Could you check a few things on this model? Use its own coordinates, in mm. A direction names the side the tool comes from. Give positions to 0.01 mm unless a question says otherwise; leave off trailing zeros. Write each loop counter-clockwise with the first axis right and the second up, starting at its lowest first coordinate (ties: lowest second). Pieces come first, ordered by that corner, then holes. Notation, with made-up numbers: (57.5, -14.75) - (90.5, -14.75) arc R13 ccw to (90.5, -4.75) - close; hole circle Ø10 at (20.5, 32). An arc over 180 degrees is marked (long way). Write item = value, one per line.
from build123d import *

# Parameters (mm, degrees)
BOSS_EXTRUDE1_DEPTH = 60
CUT_EXTRUDE3_REACH  = 29
SKETCH8_R           = 3.999999996
CUT_EXTRUDE4_REACH  = 52
SKETCH9_R           = 4.000000003
FILLET2_R           = 2


with BuildPart() as part:
    # Sketch1 → Boss-Extrude1 (new body)
    with BuildSketch(Plane(origin=(0, 0, 0), x_dir=(0, 0, -1), z_dir=(1, 0, 0))):
        Polygon((0, 0), (0, 50), (4, 50), (4, 4), (27, 4), (27, 0), align=None)
    extrude(amount=BOSS_EXTRUDE1_DEPTH)

    # Sketch8 → Cut-Extrude3 (cut, up to next)
    with BuildSketch(Plane.XY, mode=Mode.PRIVATE) as cut_extrude3_sk1:
        with Locations((10, 22)):
            Circle(SKETCH8_R)
    cut_extrude3_tool1 = extrude(cut_extrude3_sk1.sketch, amount=-CUT_EXTRUDE3_REACH, mode=Mode.PRIVATE) & part.part
    add(cut_extrude3_tool1.solids().sort_by_distance((10, 22, 0))[0], mode=Mode.SUBTRACT)
    # Sketch8 → Cut-Extrude3 (cut, up to next)
    with BuildSketch(Plane.XY, mode=Mode.PRIVATE) as cut_extrude3_sk2:
        with Locations((50, 22)):
            Circle(SKETCH8_R)
    cut_extrude3_tool2 = extrude(cut_extrude3_sk2.sketch, amount=-CUT_EXTRUDE3_REACH, mode=Mode.PRIVATE) & part.part
    add(cut_extrude3_tool2.solids().sort_by_distance((50, 22, 0))[0], mode=Mode.SUBTRACT)
    # Sketch8 → Cut-Extrude3 (cut, up to next)
    with BuildSketch(Plane.XY, mode=Mode.PRIVATE) as cut_extrude3_sk3:
        with Locations((50, 42)):
            Circle(SKETCH8_R)
    cut_extrude3_tool3 = extrude(cut_extrude3_sk3.sketch, amount=-CUT_EXTRUDE3_REACH, mode=Mode.PRIVATE) & part.part
    add(cut_extrude3_tool3.solids().sort_by_distance((50, 42, 0))[0], mode=Mode.SUBTRACT)
    # Sketch8 → Cut-Extrude3 (cut, up to next)
    with BuildSketch(Plane.XY, mode=Mode.PRIVATE) as cut_extrude3_sk4:
        with Locations((10, 42)):
            Circle(SKETCH8_R)
    cut_extrude3_tool4 = extrude(cut_extrude3_sk4.sketch, amount=-CUT_EXTRUDE3_REACH, mode=Mode.PRIVATE) & part.part
    add(cut_extrude3_tool4.solids().sort_by_distance((10, 42, 0))[0], mode=Mode.SUBTRACT)

    # Sketch9 → Cut-Extrude4 (cut, up to next)
    with BuildSketch(Plane.XZ, mode=Mode.PRIVATE) as cut_extrude4_sk1:
        with Locations((50, -19)):
            Circle(SKETCH9_R)
    cut_extrude4_tool1 = extrude(cut_extrude4_sk1.sketch, amount=-CUT_EXTRUDE4_REACH, mode=Mode.PRIVATE) & part.part
    add(cut_extrude4_tool1.solids().sort_by_distance((50, 0, -19))[0], mode=Mode.SUBTRACT)
    # Sketch9 → Cut-Extrude4 (cut, up to next)
    with BuildSketch(Plane.XZ, mode=Mode.PRIVATE) as cut_extrude4_sk2:
        with Locations((10, -19)):
            Circle(SKETCH9_R)
    cut_extrude4_tool2 = extrude(cut_extrude4_sk2.sketch, amount=-CUT_EXTRUDE4_REACH, mode=Mode.PRIVATE) & part.part
    add(cut_extrude4_tool2.solids().sort_by_distance((10, 0, -19))[0], mode=Mode.SUBTRACT)

    # Fillet2
    fillet2_edges = [part.edges().sort_by_distance(p)[0] for p in [
        (60, 50, -2),
        (0, 50, -2),
        (60, 2, -27),
        (0, 2, -27),
    ]]
    fillet(fillet2_edges, radius=FILLET2_R)


solid = part.part
1. I need wall thicknesses on line 1 (Z direction, x = 10, y = 2.4); line 2 (X direction, y = 39, z = -2.25); line 3 (Z direction, x = 37, y = 19). Which ranges of each line are inside material? Lowest first, please.
Filled sheet:
line_1 = -27 to -23, -15 to 0
line_2 = 0 to 7.35, 12.65 to 47.35, 52.65 to 60
line_3 = -4 to 0
2. For pin 1 (6.5 mm diameter, centred on x = 50, y = 22, fed in from +Z); pin 2 (11.5 mm diameter, centred on x = 35, z = -18, fed in from +Y); pin 3 (4 mm diameter, centred on x = 10.5, y = 37.5, fed in from -Z), each with a flat end and sliding along its axis, tell me the tip position at first contact or that it passes through.
Filled sheet:
pin_1 = through
pin_2 = 4
pin_3 = -4
3. Thinking about a two-plate mould opening in Z: for faces 3 (the face through (13.815, 1.972, -17.799)), 4 (the face through (60, 17, -3)), 5 (the face through (30, 25, 0)), which applies, pulls with the +Z half, pulls with the -Z half, needs draft (parallel to the pull), parting line crosses it, or undercut?
Filled sheet:
face_3 = undercut
face_4 = needs draft
face_5 = pulls with the +Z half
4. If we section it at D-D, the plane x = 33: Please give me the cut outline in (y, z).
Filled sheet:
outline = (0, -27) - (4, -27) - (4, -4) - (50, -4) - (50, 0) - (0, 0) - close
5. Which directions (+Z, -Z, +X, -X, +Y, -Y) give clear straight access to the entire face, cutting with the end or side of a thin tool? Please do faces 1 (the face through (30, 27, -4)), 2 (the face through (30, 0, -14)).
Filled sheet:
face_1 = -Z, +X, -X, +Y
face_2 = +Z, -Z, +X, -X, -Y
6. If we section it at A-A, the plane z = -19: Please give me the cut outline in (x, y), and give its area (3 significant figures).
Filled sheet:
outline = (0, 0) - (6, 0) - (6, 4) - (0, 4) - close; (14, 0) - (46, 0) - (46, 4) - (14, 4) - close; (54, 0) - (60, 0) - (60, 4) - (54, 4) - close
area = 176 mm2
7. If we section it at C-C, the plane y = 22: Please give me the cut outline in (x, z), and give its area (3 significant figures).
Filled sheet:
outline = (0, -4) - (6, -4) - (6, 0) - (0, 0) - close; (14, -4) - (46, -4) - (46, 0) - (14, 0) - close; (54, -4) - (60, -4) - (60, 0) - (54, 0) - close
area = 176 mm2
8. If we section it at B-B, the plane x = 10: Please give me the cut outline in (y, z), and give its area (3 significant figures).
Filled sheet:
outline = (0, -27) - (4, -27) - (4, -23) - (0, -23) - close; (0, -15) - (4, -15) - (4, -4) - (18, -4) - (18, 0) - (0, 0) - close; (26, -4) - (38, -4) - (38, 0) - (26, 0) - close; (46, -4) - (50, -4) - (50, 0) - (46, 0) - close
area = 196 mm2
